Build history of the part. All positions in model axes, mm. A direction names the side the tool comes from. Coordinates: 2 decimals unless noted, no trailing zeros. Order: outer loops, then holes, each group sorted by start corner. A loop starts at its lowest first (then second) coordinate and runs counter-clockwise, first axis right, second up. Notation, with made-up numbers: (8, 2) - (55, 2) arc R26 ccw to (55, 32) - close; hole circle Ø8 at (13, 66.5). An arc over 180 degrees is marked (long way). Return JSON: item names as keys, results as strings.
from build123d import *

# Parameters (mm, degrees)
ESQUISSE2_W                                   = 40
ESQUISSE2_H                                   = 10
BOSS_EXTRU_1_DEPTH                            = 40
DIAM_TRE_DU_PER_AGE_4_1_4_1_1_D               = 4.1
TROU_POUR_TARAUDAGE_POUR_TROU_TARAUD_M6_D     = 5
TROU_POUR_TARAUDAGE_POUR_TROU_TARAUD_M6_DEPTH = 8
TROU_POUR_TARAUDAGE_POUR_TROU_TARAUD_M6_TIP   = 1.502151548
DIAM_TRE_DU_PER_AGE_6_0_6_1_D                 = 6
DIAM_TRE_DU_PER_AGE_6_0_6_1_DEPTH             = 20
DIAM_TRE_DU_PER_AGE_6_0_6_1_TIP               = 1.802581857
TROU_POUR_TARAUDAGE_POUR_TROU_TARAUD_M3_D     = 2.5
TROU_POUR_TARAUDAGE_POUR_TROU_TARAUD_2_D      = 2.5
TROU_POUR_TARAUDAGE_POUR_TROU_TARAUD_2_DEPTH  = 5
TROU_POUR_TARAUDAGE_POUR_TROU_TARAUD_2_TIP    = 0.751075774
CHANFREIN1_SIZE                               = 0.5
ESQUISSE20_W                                  = 15
ESQUISSE20_H                                  = 1.6
ENL_V_MAT_EXTRU_1_DEPTH                       = 58.445626465
R_P_TITION_LIN_AIRE1_COUNT                    = 8
R_P_TITION_LIN_AIRE1_PITCH                    = 3.2


with BuildPart() as part:
    # Esquisse2 → Boss.-Extru.1 (new body)
    with BuildSketch(Plane.XY):
        with Locations((20, 5)):
            Rectangle(ESQUISSE2_W, ESQUISSE2_H)
    extrude(amount=BOSS_EXTRU_1_DEPTH)

    # Diamètre du perçage Ø4.1 (4.1)1 (through all)
    with Locations(Plane.XY.offset(40)):
        with Locations((20, 5)):
            Hole(DIAM_TRE_DU_PER_AGE_4_1_4_1_1_D / 2)

    # Trou pour taraudage pour trou taraudé M61
    with Locations(Plane.XY.offset(40)):
        with Locations((20, 5)):
            Hole(TROU_POUR_TARAUDAGE_POUR_TROU_TARAUD_M6_D / 2, depth=TROU_POUR_TARAUDAGE_POUR_TROU_TARAUD_M6_DEPTH)
            with Locations((0, 0, -(TROU_POUR_TARAUDAGE_POUR_TROU_TARAUD_M6_DEPTH + TROU_POUR_TARAUDAGE_POUR_TROU_TARAUD_M6_TIP / 2))):  # 118° drill point
                Cone(0, TROU_POUR_TARAUDAGE_POUR_TROU_TARAUD_M6_D / 2, TROU_POUR_TARAUDAGE_POUR_TROU_TARAUD_M6_TIP, mode=Mode.SUBTRACT)

    # Diamètre du perçage Ø6.0 (6)1
    with Locations(Plane(origin=(0, 0, 0), x_dir=(-1, 0, 0), z_dir=(0, 0, -1))):
        with Locations((-20, 5)):
            Hole(DIAM_TRE_DU_PER_AGE_6_0_6_1_D / 2, depth=DIAM_TRE_DU_PER_AGE_6_0_6_1_DEPTH)
            with Locations((0, 0, -(DIAM_TRE_DU_PER_AGE_6_0_6_1_DEPTH + DIAM_TRE_DU_PER_AGE_6_0_6_1_TIP / 2))):  # 118° drill point
                Cone(0, DIAM_TRE_DU_PER_AGE_6_0_6_1_D / 2, DIAM_TRE_DU_PER_AGE_6_0_6_1_TIP, mode=Mode.SUBTRACT)

    # Trou pour taraudage pour trou taraud_ M3 (through all)
    with Locations(Plane(origin=(0, 0, 0), x_dir=(-1, 0, 0), z_dir=(0, -1, 0))):
        with Locations((-4, -36), (-36, -36), (-36, -4), (-4, -4)):
            Hole(TROU_POUR_TARAUDAGE_POUR_TROU_TARAUD_M3_D / 2)

    # Trou pour taraudage pour trou taraud 2
    with Locations(Plane(origin=(0, 0, 0), x_dir=(-1, 0, 0), z_dir=(0, -1, 0))):
        with Locations((-20, -4)):
            Hole(TROU_POUR_TARAUDAGE_POUR_TROU_TARAUD_2_D / 2, depth=TROU_POUR_TARAUDAGE_POUR_TROU_TARAUD_2_DEPTH)
            with Locations((0, 0, -(TROU_POUR_TARAUDAGE_POUR_TROU_TARAUD_2_DEPTH + TROU_POUR_TARAUDAGE_POUR_TROU_TARAUD_2_TIP / 2))):  # 118° drill point
                Cone(0, TROU_POUR_TARAUDAGE_POUR_TROU_TARAUD_2_D / 2, TROU_POUR_TARAUDAGE_POUR_TROU_TARAUD_2_TIP, mode=Mode.SUBTRACT)

    # Chanfrein1
    chanfrein1_edges = [part.edges().sort_by_distance(p)[0] for p in [
        (40, 5, 40),
        (20, 10, 40),
        (0, 5, 40),
        (20, 10, 0),
        (40, 5, 0),
        (20, 0, 0),
        (0, 5, 0),
        (20, 0, 40),
        (0, 10, 20),
        (40, 10, 20),
        (40, 0, 20),
        (0, 0, 20),
    ]]
    chamfer(chanfrein1_edges, length=CHANFREIN1_SIZE)

    # Esquisse20 → Enlèv. mat.-Extru.1 (cut, through all)
    with BuildSketch(Plane(origin=(0, 0, 0), x_dir=(-1, 0, 0), z_dir=(0, -1, 0))):
        with Locations((-7.5, -31.2)):
            Rectangle(ESQUISSE20_W, ESQUISSE20_H)
        with Locations((-32.5, -31.2)):
            Rectangle(ESQUISSE20_W, ESQUISSE20_H)
    enl_v_mat_extru_1 = extrude(amount=-ENL_V_MAT_EXTRU_1_DEPTH, mode=Mode.SUBTRACT)

    # Répétition linéaire1: Enlèv. mat.-Extru.1 ×8
    with Locations(*[(0, 0, -i * R_P_TITION_LIN_AIRE1_PITCH) for i in range(1, R_P_TITION_LIN_AIRE1_COUNT)]):
        add(enl_v_mat_extru_1, mode=Mode.SUBTRACT)


solid = part.part
1. Cut at B-B on z = 4. Give the cut face in (x, y), plus the area to 3 significant figures.
Check values:
{"outline": "(0, 0.5) - (0.5, 0) - (2.75, 0) - (2.75, 10) - (0.5, 10) - (0, 9.5) - close; (5.25, 0) - (18.75, 0) - (18.75, 2.27) arc R3 cw (long way) to (21.25, 2.27) - (21.25, 0) - (34.75, 0) - (34.75, 10) - (5.25, 10) - close; (37.25, 0) - (39.5, 0) - (40, 0.5) - (40, 9.5) - (39.5, 10) - (37.25, 10) - close", "area": "316 mm²"}
2. Probe L1, parallel to X at y = 5, z = 10; L2, parallel to X at y = 5, z = 9; L3, parallel to Y at x = 20, z = 28.75. List the from-to ranges inside material, lowest first.
Check values:
{"L1": "0 to 17, 23 to 40", "L2": "15 to 17, 23 to 25", "L3": "0 to 2.95, 7.05 to 10"}
3. Drop flat-ended pins along their axis: pin 1 (0.8 mm diameter, centred on y = 6, z = 9, fed in from +X); pin 2 (0.5 mm diameter, centred on y = 6.5, z = 24.5, fed in from -X). Give the stop position or say it passes through.
Check values:
{"pin 1": "x = 25", "pin 2": "x = 15"}
4. Mould opens along Z. For faces 6 (the flat face through (8, 5, 30.4)), 7 (the flat face through (40, 5, 36)) say: pulls with the +Z half, pulls with the -Z half, needs draft (parallel to the pull), parting line crosses it, or undercut.
Check values:
{"face 6": "undercut", "face 7": "needs draft"}
5. Cut at A-A on x = 20. Give the cut face in (y, z), plus the area to 3 significant figures.
Check values:
{"outline": "(0, 0.5) - (0.5, 0) - (2, 0) - (2, 2.75) - (0, 2.75) - close; (0, 5.25) - (2, 5.25) - (2, 20) - (2.95, 20.57) - (2.95, 31.73) - (2.5, 32) - (2.5, 40) - (0.5, 40) - (0, 39.5) - close; (7.05, 20.57) - (8, 20) - (8, 0) - (9.5, 0) - (10, 0.5) - (10, 39.5) - (9.5, 40) - (7.5, 40) - (7.5, 32) - (7.05, 31.73) - close", "area": "185 mm²"}
6. Cut at C-C on z = 36. Give the cut face in (x, y).
Check values:
{"outline": "(0, 0.5) - (0.5, 0) - (2.75, 0) - (2.75, 10) - (0.5, 10) - (0, 9.5) - close; (5.25, 0) - (34.75, 0) - (34.75, 10) - (5.25, 10) - close; (37.25, 0) - (39.5, 0) - (40, 0.5) - (40, 9.5) - (39.5, 10) - (37.25, 10) - close; hole circle Ø5 at (20, 5)"}
7. Cut at D-D on y = 5. State how many separate pieces and enclosed holes the cut face has, plus the area to 3 significant figures.
Check values:
{"separate pieces": "2", "enclosed holes": "4", "area": "986 mm²"}
8. Tool access for faces 1 (the flat face through (8, 5, 19.2)), 2 (the flat face through (40, 5, 4)), 3 (the flat face through (25, 5, 9)), 4 (the flat face through (20, 10, 20)), 5 (the cylindrical face through (22.5, 5.1, 35.9)): list every direction of +Z, -Z, +X, -X, +Y, -Y with a clear straight run to the whole face (end or side of a thin tool).
Check values:
{"face 1": "-X, +Y, -Y", "face 2": "+Z, -Z, +X, +Y, -Y", "face 3": "+X, +Y, -Y", "face 4": "+Z, -Z, +X, -X, +Y", "face 5": "+Z"}
